Design review of the part built by this model. Coordinates are the model's own, in mm. A direction names the side the tool comes from. Give positions to 0.01 mm unless a question says otherwise; leave off trailing zeros. Loops run counter-clockwise (first coordinate to the right, second up) from the corner with the lowest first, then second, coordinate; pieces in that order, holes last. Notation, with made-up numbers: (-1, 1) - (8, 1) arc R20 ccw to (8, 18) - close; hole circle Ø9 at (-37.5, 11). An arc over 180 degrees is marked (long way). Put each result on its own line as item: value. Start each with the question number.
```python
from build123d import *

# Parameters (mm, degrees)
SKETCH1_W               = 203.2
SKETCH1_H               = 138.43
BOSS_EXTRUDE2_DEPTH     = 38.1
SHELL1_T                = -6.35
SKETCH2_W               = 25.4
SKETCH2_H               = 25.4
BOSS_EXTRUDE4_DEPTH     = 6.35
SKETCH3_R               = 3.175
CUT_EXTRUDE1_DEPTH      = 13.7
MIRROR4_COPY_1_SKETCH_W = 25.4
MIRROR4_COPY_1_SKETCH_H = 25.4
MIRROR4_COPY_1_DEPTH    = 6.35
MIRROR4_COPY_2_SKETCH_R = 3.175
MIRROR4_COPY_2_DEPTH    = 13.7


with BuildPart() as part:
    # Sketch1 → Boss-Extrude2 (new body)
    with BuildSketch(Plane(origin=(0, 0, 0), x_dir=(1, 0, 0), z_dir=(0, 1, 0))):
        Rectangle(SKETCH1_W, SKETCH1_H)
    extrude(amount=BOSS_EXTRUDE2_DEPTH)

    # Shell1
    shell1_openings = [part.faces().sort_by_distance(p)[0] for p in [
        (0, 38.1, 0),
    ]]
    offset(amount=SHELL1_T, openings=shell1_openings, kind=Kind.INTERSECTION)

    # Sketch2 → Boss-Extrude4 (add)
    with BuildSketch(Plane.XZ):
        with Locations((-88.9, 56.515)):
            Rectangle(SKETCH2_W, SKETCH2_H)
    boss_extrude4 = extrude(amount=BOSS_EXTRUDE4_DEPTH)

    # Sketch3 → Cut-Extrude1 (cut, through all)
    with BuildSketch(Plane(origin=(0, 6.35, 0), x_dir=(1, 0, 0), z_dir=(0, 1, 0))):
        with Locations((-88.9, -56.515)):
            Circle(SKETCH3_R)
    cut_extrude1 = extrude(amount=-CUT_EXTRUDE1_DEPTH, mode=Mode.SUBTRACT)

    # Mirror3: Boss-Extrude4, Cut-Extrude1 across plane
    add(boss_extrude4.mirror(Plane(origin=(0, 0, 0), x_dir=(0, 0, 1), z_dir=(1, 0, 0))))
    add(cut_extrude1.mirror(Plane(origin=(0, 0, 0), x_dir=(0, 0, 1), z_dir=(1, 0, 0))), mode=Mode.SUBTRACT)

    # Mirror4: Boss-Extrude4, Cut-Extrude1 across plane
    add(boss_extrude4.mirror(Plane.XY))
    add(cut_extrude1.mirror(Plane.XY), mode=Mode.SUBTRACT)

    # Mirror4 copy 1 sketch → Mirror4 copy 1 (add)
    with BuildSketch(Plane(origin=(0, 0, 0), x_dir=(-1, 0, 0), z_dir=(0, -1, 0))):
        with Locations((-88.9, 56.515)):
            Rectangle(MIRROR4_COPY_1_SKETCH_W, MIRROR4_COPY_1_SKETCH_H)
    extrude(amount=MIRROR4_COPY_1_DEPTH)

    # Mirror4 copy 2 sketch → Mirror4 copy 2 (cut, through all)
    with BuildSketch(Plane(origin=(0, 6.35, 0), x_dir=(-1, 0, 0), z_dir=(0, 1, 0))):
        with Locations((-88.9, -56.515)):
            Circle(MIRROR4_COPY_2_SKETCH_R)
    extrude(amount=-MIRROR4_COPY_2_DEPTH, mode=Mode.SUBTRACT)


solid = part.part
```
Item 1: Mouldability with a two-part tool opening along Z and no side actions: class faces 6 (the cylindrical face through (91.42, 0.089, -58.447)), 7 (the flat face through (1, 16, -69.215)), 8 (the flat face through (-101.6, 16, 1)) as pulls with the +Z half, pulls with the -Z half, needs draft (parallel to the pull), parting line crosses it, or undercut.
Item 2: For L1, parallel to Z at x = -88.9, y = 2 (3 decimals); L2, parallel to X at y = 23, z = -17; L3, parallel to Z at x = 81.5, y = 25.5 (3 decimals), list the stretches that pass through material, from the lowest coordinate up. Write a range as from..to.
Item 3: Consider section B-B (x = 88.9). State the section outline as (y, z) points (3 decimals), plus the area to 3 significant figures.
Item 4: Consider section C-C (z = 18.5). State the section outline as (x, y) points, plus the area to 3 significant figures.
Item 5: Consider section A-A (y = 23.5). State the section outline as (x, z) points (3 decimals), plus the area to 3 significant figures.
Item 6: Machinability: for faces 1 (the flat face through (-76.2, -3, -56)), 2 (the flat face through (-89, -3, 43.815)), 3 (the cylindrical face through (91.42, 0.089, 58.447)), 4 (the flat face through (-1, 0, -1)), 5 (the flat face through (-95.25, 22, 1)), which of the approach directions +Z, -Z, +X, -X, +Y, -Y give a long, thin tool a straight path to every point of the face, cutting with its end or side? Answer none if there is none.
Item 7: Consider section D-D (x = -42.5). State the section outline as (y, z) points (3 decimals).
Item 8: For P1, Ø7.5, axis at x = 88.9, z = 56.515, coming from the -Y side; P2, Ø4, axis at x = -88.9, z = 56.515, coming from the +Y side (3 decimals); P3, Ø10, axis at x = -88.9, z = -56.515, coming from the +Y side, all flat-tipped, find the tip position at first contact; note any pin that passes through.
Geometry says:
1. face 6: undercut
1. face 7: pulls with the -Z half
1. face 8: needs draft
2. L1: z = -69.215..-59.69, -53.34..53.34, 59.69..69.215
2. L2: x = -101.6..-95.25, 95.25..101.6
2. L3: z = -69.215..-62.865, 62.865..69.215
3. outline: (-6.35, -69.215) - (38.1, -69.215) - (38.1, -62.865) - (6.35, -62.865) - (6.35, -59.69) - (-6.35, -59.69) - close; (-6.35, -53.34) - (6.35, -53.34) - (6.35, 53.34) - (-6.35, 53.34) - (-6.35, 43.815) - (0, 43.815) - (0, -43.815) - (-6.35, -43.815) - close; (-6.35, 59.69) - (6.35, 59.69) - (6.35, 62.865) - (38.1, 62.865) - (38.1, 69.215) - (-6.35, 69.215) - close
3. area: 1,440 mm2
4. outline: (-101.6, 0) - (101.6, 0) - (101.6, 38.1) - (95.25, 38.1) - (95.25, 6.35) - (-95.25, 6.35) - (-95.25, 38.1) - (-101.6, 38.1) - close
4. area: 1,690 mm2
5. outline: (-101.6, -69.215) - (101.6, -69.215) - (101.6, 69.215) - (-101.6, 69.215) - close; hole (-95.25, -62.865) - (95.25, -62.865) - (95.25, 62.865) - (-95.25, 62.865) - close
5. area: 4,180 mm2
6. face 1: +Z, -Z, -Y
6. face 2: +X, -X, -Y
6. face 3: +Y, -Y
6. face 4: -Y
6. face 5: +Y
7. outline: (0, -69.215) - (38.1, -69.215) - (38.1, -62.865) - (6.35, -62.865) - (6.35, 62.865) - (38.1, 62.865) - (38.1, 69.215) - (0, 69.215) - close
8. P1: stops at y = -6.35
8. P2: passes through
8. P3: stops at y = 6.35
